Geometry check sheet. Reference: the model listing, model coordinates, mm. Coordinates: 2 decimals unless noted, no trailing zeros. Loops run counter-clockwise (first coordinate to the right, second up) from the corner with the lowest first, then second, coordinate; pieces in that order, holes last. Notation, with made-up numbers: (20, 21) - (24, 21) arc R17 ccw to (24, 32) - close; hole circle Ø6 at (82.25, 83). An arc over 180 degrees is marked (long way). Write each question's results on one line, items separated by ' | '. Start each with the question number.
(1) Mould release check, pull along X, two halves, no side actions. Record for faces 1 (the face through (87.48, 0.99, 84.67)), 2 (the face through (62, 0, -1)), 3 (the face through (-82.52, 0.99, -85.33)): pulls with the +X half, pulls with the -X half, needs draft (parallel to the pull), parting line crosses it, or undercut.
(2) Sectioned sample at D-D (x = 85). Enter the section's corners in (y, z), plus the area to 3 significant figures.
(3) Material ranges on probe 1 along Z at (x, y) = (66, 1.25); probe 2 along X at (y, z) = (0.95, 85); probe 3 along X at (y, z) = (0.7, 61), recorded low to high.
(4) Sectioned sample at B-B (x = -2). Enter the section's corners in (y, z).
(5) Sectioned sample at A-A (z = 30). Enter the section's corners in (x, y), plus the area to 3 significant figures.
(6) Sectioned sample at C-C (z = 85). Enter the section's corners in (x, y), plus the area to 3 significant figures.
from build123d import *

# Parameters (mm, degrees)
CROQUIS1_W              = 190
CROQUIS1_H              = 190
CROQUIS1_R              = 2.5
CROQUIS1_R_2            = 1.5
CROQUIS1_W_2            = 115
CROQUIS1_H_2            = 115
SALIENTE_EXTRUIR1_DEPTH = 2


with BuildPart() as part:
    # Croquis1 → Saliente-Extruir1 (new body)
    with BuildSketch(Plane(origin=(0, 0, 0), x_dir=(1, 0, 0), z_dir=(0, 1, 0))):
        Rectangle(CROQUIS1_W, CROQUIS1_H)
        with Locations(Location((-85, 85, 0), (0, 0, 270))):
            Circle(CROQUIS1_R, mode=Mode.SUBTRACT)
        with Locations(Location((85, 85, 0), (0, 0, 270))):
            Circle(CROQUIS1_R, mode=Mode.SUBTRACT)
        with Locations(Location((85, -85, 0), (0, 0, 270))):
            Circle(CROQUIS1_R, mode=Mode.SUBTRACT)
        with Locations(Location((-85, -85, 0), (0, 0, 270))):
            Circle(CROQUIS1_R, mode=Mode.SUBTRACT)
        with Locations(Location((-61, 61, 0), (0, 0, 270))):
            Circle(CROQUIS1_R_2, mode=Mode.SUBTRACT)
        with Locations(Location((66, 61, 0), (0, 0, 270))):
            Circle(CROQUIS1_R_2, mode=Mode.SUBTRACT)
        with Locations(Location((66, -61, 0), (0, 0, 270))):
            Circle(CROQUIS1_R_2, mode=Mode.SUBTRACT)
        with Locations(Location((-61, -61, 0), (0, 0, 270))):
            Circle(CROQUIS1_R_2, mode=Mode.SUBTRACT)
        Rectangle(CROQUIS1_W_2, CROQUIS1_H_2, mode=Mode.SUBTRACT)
    extrude(amount=SALIENTE_EXTRUIR1_DEPTH)


solid = part.part
Outcome:
1) face 1: undercut | face 2: needs draft | face 3: undercut
2) outline: (0, -95) - (2, -95) - (2, -87.5) - (0, -87.5) - close; (0, -82.5) - (2, -82.5) - (2, 82.5) - (0, 82.5) - close; (0, 87.5) - (2, 87.5) - (2, 95) - (0, 95) - close | area: 360 mm2
3) probe 1: z = -95 to -62.5, -59.5 to 59.5, 62.5 to 95 | probe 2: x = -95 to -87.5, -82.5 to 82.5, 87.5 to 95 | probe 3: x = -95 to -62.5, -59.5 to 64.5, 67.5 to 95
4) outline: (0, -95) - (2, -95) - (2, -57.5) - (0, -57.5) - close; (0, 57.5) - (2, 57.5) - (2, 95) - (0, 95) - close
5) outline: (-95, 0) - (-57.5, 0) - (-57.5, 2) - (-95, 2) - close; (57.5, 0) - (95, 0) - (95, 2) - (57.5, 2) - close | area: 150 mm2
6) outline: (-95, 0) - (-87.5, 0) - (-87.5, 2) - (-95, 2) - close; (-82.5, 0) - (82.5, 0) - (82.5, 2) - (-82.5, 2) - close; (87.5, 0) - (95, 0) - (95, 2) - (87.5, 2) - close | area: 360 mm2
